The model under review builds one solid part; all positions refer to its coordinate system, in mm. A direction names the side the tool comes from. Coordinates: 2 decimals unless noted, no trailing zeros. Write each loop counter-clockwise with the first axis right and the second up, starting at its lowest first coordinate (ties: lowest second). Pieces come first, ordered by that corner, then holes. Notation, with made-up numbers: (25.5, 24.25) - (44.5, 24.25) arc R18 cw to (44.5, 35.25) - close; hole circle Ø5 at (78, 20.5). An arc over 180 degrees is marked (long way). Return JSON: item names as keys, results as strings. Group by question number.
(1) We need section D-D on z = 30. State the section outline as (x, y) points.
(2) Draft analysis for pull direction X (two halves, no side actions). For faces 4 (the face through (-8.844, 15.198, 8.79)), 5 (the face through (16.8, 0, 17)), 6 (the face through (-4, 16.8, 5)), state which applies: released by +X, released by -X, zero draft, split by the parting line, or undercut.
(3) Tool access review of faces 1 (the face through (14.6, -7.5, 17.3)), 2 (the face through (-11.557, -5.332, 20.686)), 3 (the face through (4, -16.8, 5)): name each direction out of +Z, -Z, +X, -X, +Y, -Y from which nothing blocks a thin tool from reaching the whole face with its end or side.
(4) For pin 1 Ø3 at (x, y) = (2.5, -8.5) entering from +Z, flat-tipped, find the tip position at first contact; note if it passes through.
(5) We need section C-C on x = -10.5. State the section outline as (y, z) points.
(6) We need section A-A on y = 14.5. State the section outline as (x, z) points, then the cut area to 3 significant figures.
(7) We need section B-B on z = 12. State the section outline as (x, y) points, then the cut area to 3 significant figures.
(8) To check wall thickness, follow L1, parallel to X at y = 14.55, z = 16.9; L2, parallel to X at y = 13, z = 7; L3, parallel to Z at x = -0.5, y = -13.5. State the ranges of each line that lie inside material, in increasing order. Write a range as from..to.
Autodesk Inventor part; units mm, degrees
ref_plane "Work Plane2" through (-27.39, -0.0644, 16.8356) normal (0, -0.7071, -0.7071) x (0, 0.7071, -0.7071)
ref_plane "Work Plane3" through (-16.9, 21.1423, 33.8) normal (0, 0, -1) x (0, 1, 0)
ref_plane "YZ Plane" through (0, 0, 0) normal (1, 0, 0) x (0, 1, 0)
sketch "Sketch1" plane through (0, 0, 0) normal (0, 0, 1) x (1, 0, 0)
  line L0 (-34.86, 0) -> (34.86, 0) construction
  line L1 (0, -34.86) -> (0, 34.86) construction
  line L2 (0, 0) -> (16.9726, 16.9726) construction
  line L3 (0, 0) -> (24.0028, 0) construction
  line L4 (0, 24.9) -> (16.8009, 24.9)
  line L5 (16.8009, 24.9) -> (16.8009, 21.2415)
  line L6 (16.8009, 21.2415) -> (19.0212, 19.0212)
  line L7 (24.9, 0) -> (24.9, 16.8009)
  line L8 (24.9, 16.8009) -> (21.2415, 16.8009)
  line L9 (21.2415, 16.8009) -> (19.0212, 19.0212)
  line L10 (0, -24.9) -> (16.8009, -24.9)
  line L11 (16.8009, -24.9) -> (16.8009, -21.2415)
  line L12 (16.8009, -21.2415) -> (19.0212, -19.0212)
  line L13 (24.9, 0) -> (24.9, -16.8009)
  line L14 (24.9, -16.8009) -> (21.2415, -16.8009)
  line L15 (21.2415, -16.8009) -> (19.0212, -19.0212)
  line L16 (0, 0) -> (-16.9726, 16.9726) construction
  line L17 (0, 0) -> (-24.0028, 0) construction
  line L18 (0, 24.9) -> (-16.8009, 24.9)
  line L19 (-16.8009, 24.9) -> (-16.8009, 21.2415)
  line L20 (-16.8009, 21.2415) -> (-19.0212, 19.0212)
  line L21 (-24.9, 0) -> (-24.9, 16.8009)
  line L22 (-24.9, 16.8009) -> (-21.2415, 16.8009)
  line L23 (-21.2415, 16.8009) -> (-19.0212, 19.0212)
  line L24 (0, -24.9) -> (-16.8009, -24.9)
  line L25 (-16.8009, -24.9) -> (-16.8009, -21.2415)
  line L26 (-16.8009, -21.2415) -> (-19.0212, -19.0212)
  line L27 (-21.2415, -16.8009) -> (-19.0212, -19.0212)
  line L28 (-24.9, -16.8009) -> (-21.2415, -16.8009)
  line L29 (-24.9, 0) -> (-24.9, -16.8009)
  circle A0 centre (0, 0) radius 7.5
  dimension "d17" = 45
  dimension "d18" = 24.9
  dimension "d20" = 3.14
  dimension "d21" = 26.9
  dimension "d22" = 15
extrude "Extrusion1" add sketch "Sketch1" along normal blind 3 contours L4 L5 L6 L9 L8 L7 L13 L14 L15 L12 L11 L10 L24 L25 L26 L27 L28 L29 L21 L22 L23 L20 L19 L18 | A0
sketch "Sketch6" plane through (0, 0, 3) normal (0, 0, 1) x (1, 0, 0)
  line L0 (16.8009, 24.9) -> (-16.8009, 24.9)
  line L1 (-16.8009, 24.9) -> (-16.8009, 21.2415)
  line L2 (-16.8009, 21.2415) -> (-21.2415, 16.8009)
  line L3 (-21.2415, 16.8009) -> (-24.9, 16.8009)
  line L4 (-24.9, 16.8009) -> (-24.9, -16.8009)
  line L5 (-24.9, -16.8009) -> (-21.2415, -16.8009)
  line L6 (-21.2415, -16.8009) -> (-16.8009, -21.2415)
  line L7 (-16.8009, -21.2415) -> (-16.8009, -24.9)
  line L8 (-16.8009, -24.9) -> (16.8009, -24.9)
  line L9 (16.8009, -24.9) -> (16.8009, -21.2415)
  line L10 (16.8009, -21.2415) -> (21.2415, -16.8009)
  line L11 (21.2415, -16.8009) -> (24.9, -16.8009)
  line L12 (24.9, -16.8009) -> (24.9, 16.8009)
  line L13 (24.9, 16.8009) -> (21.2415, 16.8009)
  line L14 (21.2415, 16.8009) -> (16.8009, 21.2415)
  line L15 (16.8009, 21.2415) -> (16.8009, 24.9)
  line L16 (24.9, -16.8009) -> (24.9, 16.8009)
  line L17 (24.9, 13.5502) -> (-24.9, 13.5502)
  line L18 (-24.9, 16.8009) -> (-24.9, -16.8009)
  point P0 (0, 0)
ref_plane "Work Plane2" through (-27.39, -0.0644, 16.8356) normal (0, -0.7071, -0.7071) x (0, 0.7071, -0.7071)
extrude "Extrusion6" add sketch "Sketch6" along normal up to surface contours L12 L11 L10 L9 L8 L7 L6 L5 L4 L17 surface through (-27.39, -0.0644, 16.8356) normal (0, -0.7071, -0.7071)
sketch "Sketch7" plane through (-16.8009, -24.9, 0) normal (0, -1, 0) x (1, 0, 0)
  line L0 (-0.0991, 33.8) -> (0.8009, 33.8)
  arc A0 (-6.0991, 41.8) -> (-8.0991, 39.8) centre (-6.0991, 39.8) ccw
  arc A1 (41.7009, 39.8) -> (39.7009, 41.8) centre (39.7009, 39.8) ccw
  line L1 (41.9057, 41.8) -> (-10.6447, 41.8)
  line L2 (-10.6447, 41.8) -> (-10.6447, 33.8)
  line L3 (-10.6447, 33.8) -> (41.9057, 33.8)
  line L4 (41.9057, 33.8) -> (41.9057, 41.8)
  point P0 (16.8009, 0)
extrude "Extrusion7" cut sketch "Sketch7" against normal through all
sketch "Sketch8" plane through (21.2415, -16.8009, 0) normal (0, -1, 0) x (1, 0, 0)
  line L0 (-8.7415, 0) -> (-33.7415, 0)
  line L1 (-33.7415, -1) -> (-8.7415, -1)
  line L2 (-46.1415, 33.572) -> (-42.483, 33.572)
  line L3 (3.6585, 33.8) -> (0.0423, 33.8)
  line L4 (0, 33.572) -> (3.6585, 33.572)
  line L5 (-46.1415, 3.2209) -> (-46.1415, 33.572)
  line L6 (3.6585, 33.572) -> (-46.1415, 33.572)
  line L7 (-46.1415, 33.572) -> (-46.1415, 30.572)
  line L8 (-46.1415, 30.572) -> (3.6585, 30.572)
  line L9 (3.6585, 30.572) -> (3.6585, 33.572)
  dimension "d45" = 3
sketch "Sketch9" plane through (-16.8009, -24.9, 0) normal (0, -1, 0) x (1, 0, 0)
  line L0 (33.7009, 0) -> (33.0009, 0) construction
  line L1 (36.0327, -6) -> (22.7009, -6) construction
  circle A0 centre (16.8009, 16.9) radius 16.9 construction
  circle A1 centre (16.8009, 16.9) radius 7.5
  line L2 (39.7009, 8.1978) -> (33.7009, 8.1978)
  line L3 (33.7009, 8.1978) -> (33.7009, 0)
  line L4 (33.0009, 0) -> (33.0009, -3.7)
  line L5 (33.0009, -3.7) -> (22.7009, -3.7)
  line L6 (22.7009, -3.7) -> (22.7009, -6)
  arc A2 (39.7009, -2.3319) -> (36.0327, -6) centre (36.8009, -3.1) ccw
  line L7 (39.7009, 8.1978) -> (39.7009, -2.3319)
  point P0 (16.8009, 0)
  dimension "d46" = 15
extrude "Extrusion8" cut sketch "Sketch9" against normal through all
sketch "Sketch10" plane through (-16.8009, -24.9, 0) normal (0, -1, 0) x (1, 0, 0)
  circle A0 centre (16.8009, 16.9) radius 7.5
  circle A1 centre (16.8009, 16.9) radius 12.75
  point P0 (16.8009, 0)
  dimension "d49" = 25.5
extrude "Extrusion9" cut sketch "Sketch10" against normal blind 7
sketch "Sketch12" plane through (-24.9, 13.5502, 3.2209) normal (0, 0.7071, 0.7071) x (1, 0, 0)
  line L0 (32.9, -31.2053) -> (32.9, -6.2053) construction
  line L1 (32.9, -6.2053) -> (16.9, -6.2053) construction
  line L2 (16.9, -6.2053) -> (16.9, -31.2053) construction
  line L3 (16.9, -31.2053) -> (32.9, -31.2053) construction
  line L4 (37.7, -37.554) -> (12.1, -37.554)
  line L5 (12.1, -37.554) -> (12.1, -0.954)
  line L6 (12.1, -0.954) -> (37.7, -0.954)
  line L7 (37.7, -0.954) -> (37.7, -37.554)
  line L8 (37.7, -37.554) -> (12.1, -0.954) construction
  line L9 (12.1, -37.554) -> (37.7, -0.954) construction
  line L10 (10.6, -39.054) -> (39.2, -39.054)
  line L11 (39.2, -39.054) -> (39.2, 0.546)
  line L12 (39.2, 0.546) -> (10.6, 0.546)
  line L13 (10.6, 0.546) -> (10.6, -39.054)
  point P0 (24.9, -19.254)
  point P1 (24.9, -8.7385)
  point P2 (24.9, -8.7385)
  dimension "d81" = 25.6
  dimension "d82" = 36.6
  dimension "d83" = 1.5
sketch "Sketch13" plane through (0, 0, 3) normal (0, 0, 1) x (1, 0, 0)
  line L0 (24.9, 13.5502) -> (24.9, 16.8009)
  line L1 (24.9, 16.8009) -> (21.2415, 16.8009)
  line L2 (21.2415, 16.8009) -> (16.8009, 21.2415)
  line L3 (16.8009, 21.2415) -> (16.8009, 24.9)
  line L4 (16.8009, 24.9) -> (-16.8009, 24.9)
  line L5 (-16.8009, 24.9) -> (-16.8009, 21.2415)
  line L6 (-16.8009, 21.2415) -> (-21.2415, 16.8009)
  line L7 (-21.2415, 16.8009) -> (-24.9, 16.8009)
  line L8 (-24.9, 16.8009) -> (-24.9, 13.5502)
  line L9 (-24.9, 13.5502) -> (24.9, 13.5502)
  point P0 (0, 0)
ref_plane "Work Plane3" through (-16.9, 21.1423, 33.8) normal (0, 0, -1) x (0, 1, 0)
extrude "Extrusion12" add sketch "Sketch13" along normal up to surface (30.8 mm away)
sketch "Sketch14" plane through (-16.8009, 24.9, 0) normal (0, 1, 0) x (1, 0, 0)
  line L0 (-0.0991, -33.8) -> (-0.0991, 0) construction
  line L1 (33.6017, -33.8) -> (0, -33.8)
  line L2 (0, 0) -> (33.6017, 0)
  line L3 (33.6017, 0) -> (33.6017, -33.8)
  arc A0 (16.8009, -9.4) -> (16.8009, -9.4) centre (16.8009, -16.9) ccw construction
  circle A1 centre (16.8009, -16.9) radius 12.75
  point P0 (16.8009, 0)
  dimension "d61" = 25.5
extrude "Extrusion13" cut sketch "Sketch14" against normal blind 7
sketch "Sketch15" plane through (0, 17.9, 16.9) normal (0, 1, 0) x (1, 0, 0)
  circle A0 centre (0, 0) radius 7.5
  circle A1 centre (0, 0) radius 12
  point P0 (0, 16.9)
  dimension "d84" = 24
extrude "Extrusion14" cut sketch "Sketch15" against normal through all contours A0 | A1
sketch "Sketch16" plane through (21.2415, -16.8009, 33.572) normal (0, 0.7071, 0.7071) x (1, 0, 0)
  line L0 (-42.255, -0.3224) -> (-0.228, -0.3224)
  line L1 (-0.228, -0.3224) -> (0, 0)
  line L2 (0, 0) -> (3.6585, 0)
  line L3 (3.6585, 0) -> (3.6585, 42.9229)
  line L4 (-46.1415, 42.9229) -> (-46.1415, 0)
  line L5 (-46.1415, 0) -> (-42.483, 0)
  line L6 (-42.483, 0) -> (-42.255, -0.3224)
  line L7 (-4.4406, 18.0121) -> (-38.0423, 18.0121)
  circle A0 centre (-37.2415, 18.0121) radius 1.4
  circle A1 centre (-5.2415, 18.0121) radius 1.4
  line L8 (3.6585, 42.9229) -> (-46.1415, 42.9229)
  ellipse E0 centre (-21.2415, 23.5778) end of major axis (-21.2415, 40.5484) minor radius 12
  point P0 (-21.2415, 35.619)
  dimension "d68" = 2.8
  dimension "d69" = 2.8
  dimension "d85" = 16
extrude "Extrusion15" cut sketch "Sketch16" against normal blind 10 contours A0 | A1
sketch "Sketch17" plane through (-24.9, -16.8009, 0) normal (-1, 0, 0) x (0, 0, 1)
  line L0 (43.2726, 50.002) -> (33.5, 50.002)
  line L1 (33.5, 50.002) -> (33.5, -21.818)
  line L2 (33.5, -21.818) -> (43.2726, -21.818)
  line L3 (43.2726, -21.818) -> (43.2726, 50.002)
  line L4 (0, 0) -> (0, 33.6017)
  point P0 (0, 16.8009)
  dimension "d72" = 33.5
extrude "Extrusion16" cut sketch "Sketch17" against normal through all
ref_plane "Work Plane4" through (-12.8, -13.0045, 29.7756) normal (0, 0.7071, 0.7071) x (1, 0, 0)
sketch "Sketch19" plane through (-12.8, -13.0045, 29.7756) normal (0, 0.7071, 0.7071) x (1, 0, 0)
  line L0 (0, 36.554) -> (-1.5, 36.554)
  line L1 (-1.5, 36.554) -> (-1.5, -1.5)
  line L2 (-1.5, -1.5) -> (27.1, -1.5)
  line L3 (27.1, -1.5) -> (27.1, 36.554)
  line L4 (27.1, 36.554) -> (25.6, 36.554)
  line L5 (25.6, 36.554) -> (25.6, 0)
  line L6 (25.6, 0) -> (0, 0)
  line L7 (0, 0) -> (0, 36.554)
  line L8 (25.6, 0) -> (25.6, 36.6)
  line L9 (0, 0) -> (25.6, 0)
  line L10 (0, 36.6) -> (0, 0)
  line L11 (25.6, -1.5) -> (0, -1.5)
  line L12 (0, -1.5) -> (0, 36.6)
  line L13 (0, 36.6) -> (25.6, 36.6)
  line L14 (25.6, 36.6) -> (25.6, -1.5)
  line L15 (25.6, -1.5) -> (0, -1.5)
  line L16 (0, -1.5) -> (0, -6.2491)
  line L17 (0, -6.2491) -> (25.6, -6.2491)
  line L18 (25.6, -6.2491) -> (25.6, -1.5)
  point P0 (12.8, 30.2501)
extrude "Extrusion18" cut sketch "Sketch19" along normal mid plane 2 contours L10 L13 L8 L5 L6 L7 | L6 L14 L2 L12 | L2 L18 L17 L16
sketch "Sketch21" plane through (0, 0, 0) normal (0, 0, -1) x (-1, 0, 0)
  line L0 (16.8009, -24.9) -> (16.8009, -21.2415)
  line L1 (16.8009, -21.2415) -> (21.2415, -16.8009)
  line L2 (21.2415, -16.8009) -> (24.9, -16.8009)
  line L3 (24.9, -16.8009) -> (24.9, 16.8009)
  line L4 (24.9, 16.8009) -> (21.2415, 16.8009)
  line L5 (21.2415, 16.8009) -> (16.8009, 21.2415)
  line L6 (16.8009, 21.2415) -> (16.8009, 24.9)
  line L7 (16.8009, 24.9) -> (-16.8009, 24.9)
  line L8 (-16.8009, 24.9) -> (-16.8009, 21.2415)
  line L9 (-16.8009, 21.2415) -> (-21.2415, 16.8009)
  line L10 (-21.2415, 16.8009) -> (-24.9, 16.8009)
  line L11 (-24.9, 16.8009) -> (-24.9, -16.8009)
  line L12 (-24.9, -16.8009) -> (-21.2415, -16.8009)
  line L13 (-21.2415, -16.8009) -> (-16.8009, -21.2415)
  line L14 (-16.8009, -21.2415) -> (-16.8009, -24.9)
  line L15 (-16.8009, -24.9) -> (16.8009, -24.9)
  line L16 (-16.8, -16.8) -> (16.8, -16.8)
  line L17 (16.8, -16.8) -> (16.8, 16.8)
  line L18 (16.8, 16.8) -> (-16.8, 16.8)
  line L19 (-16.8, 16.8) -> (-16.8, -16.8)
  line L20 (-16.8, -16.8) -> (16.8, 16.8) construction
  line L21 (16.8, -16.8) -> (-16.8, 16.8) construction
  point P0 (0, 0)
  point P1 (0, 0)
  dimension "d92" = 33.6
  dimension "d93" = 33.6
extrude "Extrusion20" cut sketch "Sketch21" against normal through all contours L19 L18 L17 L16 keep common part
sketch "Sketch22" plane through (-16.8, 16.8, 33.5) normal (0, 0, 1) x (1, 0, 0)
  line L0 (33.6, -33.5288) -> (33.6, -33.6)
  line L1 (0, 0) -> (33.6, 0)
  line L2 (0, -33.6) -> (0, -33.5288)
  line L3 (41.7, -33.6009) -> (-8.1, -33.6009)
  line L4 (33.6, 0) -> (33.6, -33.6)
  line L5 (29.6, -33.5288) -> (33.6, -33.5288)
  line L6 (33.6, 0) -> (31.6, 0)
  line L7 (31.6, 0) -> (31.6, -33.5288)
  line L8 (31.6, -33.5288) -> (33.6, -33.5288)
  line L9 (33.6, -33.5288) -> (33.6, 0)
  line L10 (33.6, 0) -> (0, 0)
  line L11 (0, -33.5288) -> (4, -33.5288)
  line L12 (0, 0) -> (2, 0)
  line L13 (2, 0) -> (2, -33.5288)
  line L14 (2, -33.5288) -> (0, -33.5288)
  line L15 (0, -33.5288) -> (0, 0)
  line L16 (33.6, -33.6) -> (29.6, -33.6)
  line L17 (4, -33.6) -> (0, -33.6)
  line L18 (4, -33.6) -> (4, -33.5288)
  line L19 (29.6, -33.5288) -> (29.6, -33.6)
  line L20 (29.6, -33.5288) -> (33.6, -33.5288)
  line L21 (33.6, 0) -> (33.6, -3.2498)
  line L22 (0, -3.2498) -> (0, 0)
  line L23 (33.6, -3.2498) -> (0, -3.2498)
  line L24 (0, -33.5288) -> (4, -33.5288)
  point P0 (16.8, -16.8)
  point P1 (33.6, -3.2498)
  point P2 (2, 0)
extrude "Extrusion21" add sketch "Sketch22" against normal up to surface (33.5 mm away) contours L5 L7 L23 L4 | L23 L7 L1 L4 | L3 L2 L11 L18 | L23 L15 L1 L13 | L13 L11 L15 L23
properties part number "20_Cube_Insert_Beamsplittercube_Base_25x35_v3"
Ans:
{
 "1": {"outline": "(-16.8, -16.8) - (16.8, -16.8) - (16.8, 16.8) - (-16.8, 16.8) - close; hole (-14.8, -13.23) - (-12.8, -13.23) - (-12.8, -14.65) - (12.8, -14.65) - (12.8, -13.23) - (14.8, -13.23) - (14.8, 13.55) - (-14.8, 13.55) - close"},
 "2": {"face 4": "undercut", "face 5": "released by +X", "face 6": "zero draft"},
 "3": {"face 1": "none", "face 2": "+Z", "face 3": "+Z, -Z, +X, -X, -Y"},
 "4": {"pin 1": "z = 5.59"},
 "5": {"outline": "(-16.8, 0) - (16.8, 0) - (16.8, 11.09) - (13.55, 11.09) - (13.55, 4.64) - (13.58, 4.6) - (13.55, 4.57) - (13.55, 3.22) - (12.88, 3.9) - (12.17, 3.19) - (4.26, 11.09) - (-16.8, 11.09) - close; (-16.8, 22.71) - (-7.36, 22.71) - (-16.8, 32.15) - close; (13.55, 22.71) - (16.8, 22.71) - (16.8, 33.5) - (13.55, 33.5) - close"},
 "6": {"outline": "(-16.8, 0) - (16.8, 0) - (16.8, 33.5) - (-16.8, 33.5) - close; hole circle Ø24 at (0, 16.9)", "area": "673 mm²"},
 "7": {"outline": "(-16.8, -16.8) - (-10.95, -16.8) - (-10.95, 3.35) - (-12.8, 3.35) - (-12.8, 4.77) - (-14.8, 4.77) - (-14.8, 13.55) - (-10.95, 13.55) - (-10.95, 16.8) - (-16.8, 16.8) - close; (10.95, -16.8) - (16.8, -16.8) - (16.8, 16.8) - (10.95, 16.8) - (10.95, 13.55) - (14.8, 13.55) - (14.8, 4.77) - (12.8, 4.77) - (12.8, 3.35) - (10.95, 3.35) - close", "area": "320 mm²"},
 "8": {"L1": "-16.8..-12, 12..16.8", "L2": "-16.8..-14.8, 14.8..16.8", "L3": "0..4.91"}
}
